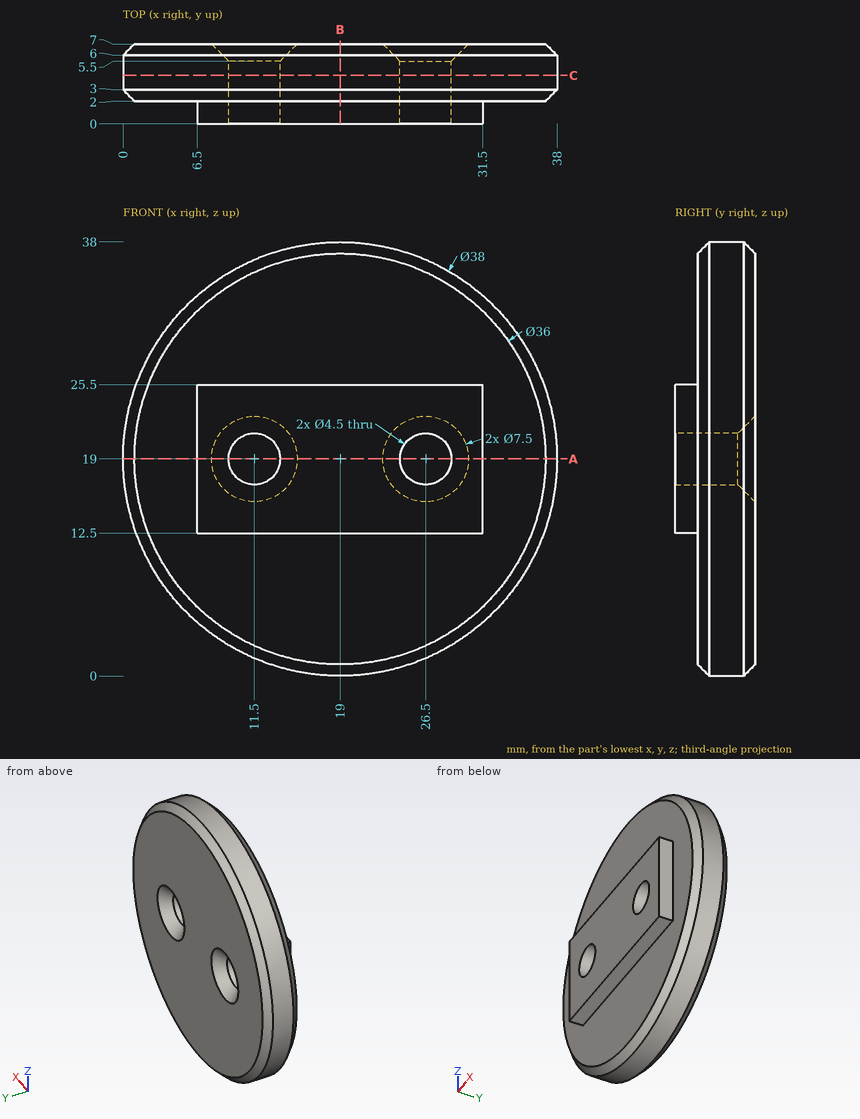
Answer from the drawing. Dimensions are ordinates in mm from the lowest x, y and z of the part. Coordinates: 2 decimals unless noted, no trailing zeros. Loops run counter-clockwise (first coordinate to the right, second up) from the corner with the lowest first, then second, coordinate; pieces in that order, holes last. Notation, with made-up numbers: (-18.75, 66.25) -> (11.25, 66.25) arc R18 cw to (11.25, 71.25) -> close; hole circle Ø2 at (74.5, 55.5). An arc over 180 degrees is marked (long way). Answer in a Markdown table with one row per item.
Item 1: A cutting plane is placed at A-A on z = 19. Determine the outline of the cut face in (x, y).
Returned:
| item | result |
|---|---|
| outline | (0, 3) -> (1, 2) -> (6.5, 2) -> (6.5, 0) -> (9.25, 0) -> (9.25, 5.5) -> (7.75, 7) -> (1, 7) -> (0, 6) -> close; (13.75, 0) -> (24.25, 0) -> (24.25, 5.5) -> (22.75, 7) -> (15.25, 7) -> (13.75, 5.5) -> close; (28.75, 0) -> (31.5, 0) -> (31.5, 2) -> (37, 2) -> (38, 3) -> (38, 6) -> (37, 7) -> (30.25, 7) -> (28.75, 5.5) -> close |
Item 2: Straight lines are drawn through the part: line 1 along X through (y, z) = (4.2, 19); line 2 along X through (y, z) = (1.55, 19); line 3 along Y through (x, z) = (24, 5.5). For each, find the intervals that lie inside material, in ascending order. Write a range as [from, to].
Returned:
| item | result |
|---|---|
| line 1 | x = [0, 9.25], [13.75, 24.25], [28.75, 38] |
| line 2 | x = [6.5, 9.25], [13.75, 24.25], [28.75, 31.5] |
| line 3 | y = [2, 7] |
Item 3: A cutting plane is placed at C-C on y = 4.25. Determine the outline of the cut face in (x, z), plus the area to 3 significant figures.
Returned:
| item | result |
|---|---|
| outline | circle Ø38 at (19, 19); hole circle Ø4.5 at (11.5, 19); hole circle Ø4.5 at (26.5, 19) |
| area | 1,100 mm^2 |
Item 4: Each of these flat-tipped pins is pushed along its axis until it touches: P1, Ø1, axis at y = 1, z = 18, coming from the +X side; P2, Ø4, axis at x = 23, y = 6, coming from the +Z side; P3, Ø0.6, axis at y = 1.5, z = 17.5, coming from the -X side; P4, Ø4, axis at x = 13, z = 15.5, coming from the -Y side. Where does it stop, or does it pass through?
Returned:
| item | result |
|---|---|
| P1 | stops at x = 31.5 |
| P2 | stops at z = 37.89 |
| P3 | stops at x = 6.5 |
| P4 | stops at y = 0 |
Item 5: A cutting plane is placed at B-B on x = 19. Determine the outline of the cut face in (y, z).
Returned:
| item | result |
|---|---|
| outline | (0, 12.5) -> (2, 12.5) -> (2, 1) -> (3, 0) -> (6, 0) -> (7, 1) -> (7, 37) -> (6, 38) -> (3, 38) -> (2, 37) -> (2, 25.5) -> (0, 25.5) -> close |
